```python
from build123d import *

# Parameters (mm, degrees)
SKETCH1_W           = 50
SKETCH1_H           = 15.25
SKETCH1_W_2         = 2
SKETCH1_H_2         = 5
SKETCH1_W_3         = 7
SKETCH1_H_3         = 2
BOSS_EXTRUDE1_DEPTH = 2


with BuildPart() as part:
    # Sketch1 → Boss-Extrude1 (new body)
    # profile 1 of 7: a face of its own
    with BuildSketch(Plane(origin=(0, 0, 0), x_dir=(0, 0, -1), z_dir=(1, 0, 0))):
        Rectangle(SKETCH1_W, SKETCH1_H)
        with Locations((-9, -0.125)):
            Rectangle(SKETCH1_W_2, SKETCH1_H_2, mode=Mode.SUBTRACT)
        with Locations((9, -0.125)):
            Rectangle(SKETCH1_W_2, SKETCH1_H_2, mode=Mode.SUBTRACT)
        with Locations((-13, 0.125)):
            Rectangle(SKETCH1_W_2, SKETCH1_H_2, mode=Mode.SUBTRACT)
        with Locations((13, 0.125)):
            Rectangle(SKETCH1_W_2, SKETCH1_H_2, mode=Mode.SUBTRACT)
    # profile 2 of 7: a face of its own
    with BuildSketch(Plane(origin=(0, 0, 0), x_dir=(0, 0, -1), z_dir=(1, 0, 0))):
        with Locations((-15.5, -8.625)):
            Rectangle(SKETCH1_W_3, SKETCH1_H_3)
    # profile 3 of 7: a face of its own
    with BuildSketch(Plane(origin=(0, 0, 0), x_dir=(0, 0, -1), z_dir=(1, 0, 0))):
        with Locations((0, -8.625)):
            Rectangle(SKETCH1_W_3, SKETCH1_H_3)
    # profile 4 of 7: a face of its own
    with BuildSketch(Plane(origin=(0, 0, 0), x_dir=(0, 0, -1), z_dir=(1, 0, 0))):
        with Locations((15.5, -8.625)):
            Rectangle(SKETCH1_W_3, SKETCH1_H_3)
    # profile 5 of 7: a face of its own
    with BuildSketch(Plane(origin=(0, 0, 0), x_dir=(0, 0, -1), z_dir=(1, 0, 0))):
        with Locations((-15.5, 8.625)):
            Rectangle(SKETCH1_W_3, SKETCH1_H_3)
    # profile 6 of 7: a face of its own
    with BuildSketch(Plane(origin=(0, 0, 0), x_dir=(0, 0, -1), z_dir=(1, 0, 0))):
        with Locations((0, 8.625)):
            Rectangle(SKETCH1_W_3, SKETCH1_H_3)
    # profile 7 of 7: a face of its own
    with BuildSketch(Plane(origin=(0, 0, 0), x_dir=(0, 0, -1), z_dir=(1, 0, 0))):
        with Locations((15.5, 8.625)):
            Rectangle(SKETCH1_W_3, SKETCH1_H_3)
    extrude(amount=BOSS_EXTRUDE1_DEPTH)


solid = part.part
```
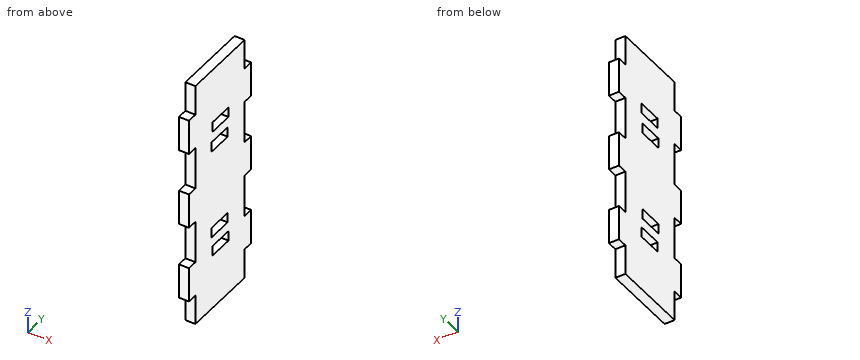
Check sheet for the modelled part. Datum: model origin and axes. Units: mm. Give positions to 0.01 mm unless a question says otherwise; leave off trailing zeros. Order: outer loops, then holes, each group sorted by start corner. A loop starts at its lowest first (then second) coordinate and runs counter-clockwise, first axis right, second up. Notation, with made-up numbers: (19, 71.25) -> (33, 71.25) arc R28 cw to (33, 101.25) -> close; hole circle Ø8 at (1.5, 51.25). An arc over 180 degrees is marked (long way). Return JSON: item names as keys, results as strings.
1. Cross-section at A-A, the plane y = 0. Record the cut outline in (x, z), plus the area to 3 significant figures.
From the geometry:
{"outline": "(0, -25) -> (2, -25) -> (2, -14) -> (0, -14) -> close; (0, -12) -> (2, -12) -> (2, -10) -> (0, -10) -> close; (0, -8) -> (2, -8) -> (2, 8) -> (0, 8) -> close; (0, 10) -> (2, 10) -> (2, 12) -> (0, 12) -> close; (0, 14) -> (2, 14) -> (2, 25) -> (0, 25) -> close", "area": "84.0 mm^2"}
2. Cross-section at C-C, the plane x = 0.3. Count the separate pieces of the cut face and the enclosed holes in it, plus the area to 4 significant figures.
From the geometry:
{"separate pieces": "1", "enclosed holes": "4", "area": "806.5 mm^2"}
3. Cross-section at B-B, the plane y = -8.5. Record the cut outline in (x, z), plus the area to 3 significant figures.
From the geometry:
{"outline": "(0, -19) -> (2, -19) -> (2, -12) -> (0, -12) -> close; (0, -3.5) -> (2, -3.5) -> (2, 3.5) -> (0, 3.5) -> close; (0, 12) -> (2, 12) -> (2, 19) -> (0, 19) -> close", "area": "42.0 mm^2"}
4. Material ranges on probe 1 along Z at (x, y) = (0.2, -1.25); probe 2 along Z at (x, y) = (1.8, 7.75); probe 3 along Y at (x, z) = (1.5, 20) (3 decimals), recorded low to high. Write a range as [from, to].
From the geometry:
{"probe 1": "[-25, -14], [-12, -10], [-8, 8], [10, 12], [14, 25]", "probe 2": "[-19, -12], [-3.5, 3.5], [12, 19]", "probe 3": "[-7.625, 7.625]"}
5. Go/stop test with flat-tipped pins: P1, Ø1, axis at x = 1, z = 21, coming from the +Y side (3 decimals); P2, Ø1, axis at x = 0.5, y = -8.5, coming from the -Z side; P3, Ø1, axis at x = 1.5, y = -8.5, coming from the +Z side. Record where each tip stops, or that it passes through.
From the geometry:
{"P1": "y = 7.625", "P2": "z = -19", "P3": "z = 19"}
